The model under review builds one solid part; all positions refer to its coordinate system, in mm. A direction names the side the tool comes from. Round coordinates to 2 decimals unless told otherwise and drop trailing zeros. Write each loop counter-clockwise with the first axis right and the second up, starting at its lowest first coordinate (ties: lowest second). Pieces come first, ordered by that corner, then holes. Notation, with made-up numbers: (25.5, 3.25) - (48.5, 3.25) arc R9 ccw to (48.5, 16.25) - close; hole circle Ø9 at (50, 45). An arc over 180 degrees is marked (long way). Use one line per item in the form item = value.
from build123d import *

# Parameters (mm, degrees)
SKETCH1_W           = 7
SKETCH1_H           = 7
BOSS_EXTRUDE1_DEPTH = 3
CUT_EXTRUDE1_DEPTH  = 7
CUT_EXTRUDE2_DEPTH  = 11
SKETCH4_R           = 1.8
CUT_EXTRUDE3_DEPTH  = 0.8
CUT_EXTRUDE4_DEPTH  = 0.4


with BuildPart() as part:
    # Sketch1 → Boss-Extrude1 (new body)
    with BuildSketch(Plane(origin=(0, 0, 0), x_dir=(1, 0, 0), z_dir=(0, 1, 0))):
        with Locations((3.5, 3.5)):
            Rectangle(SKETCH1_W, SKETCH1_H)
    extrude(amount=BOSS_EXTRUDE1_DEPTH)

    # Sketch2 → Cut-Extrude1 (cut)
    with BuildSketch(Plane.XY):
        Polygon((0, 0), (0.7, 3), (0, 3), align=None)
        Polygon((7, 0), (6.3, 3), (7, 3), align=None)
    extrude(amount=-CUT_EXTRUDE1_DEPTH, mode=Mode.SUBTRACT)

    # Sketch3 → Cut-Extrude2 (cut)
    with BuildSketch(Plane(origin=(0, 0, 0), x_dir=(0, 0, -1), z_dir=(1, 0, 0))):
        Polygon((0, 0), (0.7, 3), (0, 3), align=None)
        Polygon((7, 3), (6.3, 3), (7, 0), align=None)
    extrude(amount=CUT_EXTRUDE2_DEPTH, mode=Mode.SUBTRACT)

    # Sketch4 → Cut-Extrude3 (cut)
    with BuildSketch(Plane.XZ):
        with Locations(Location((3.5, -3.5, 0), (0, 0, 270))):
            Circle(SKETCH4_R)
    extrude(amount=-CUT_EXTRUDE3_DEPTH, mode=Mode.SUBTRACT)

    # Sketch5 → Cut-Extrude4 (cut)
    with BuildSketch(Plane(origin=(0, 3, 0), x_dir=(1, 0, 0), z_dir=(0, 1, 0))):
        with BuildLine():
            Line((2.273436966, 1.766029319), (2.273436966, 5.266029319))
            Line((2.273436966, 5.266029319), (3.393128472, 5.266029319))
            add(Edge.make_bspline(
                [(3.393128472, 5.266029319), (3.443844607, 5.265973935), (3.540845243, 5.265868005), (3.679210782, 5.262924846), (3.803788221, 5.25875848), (3.914392667, 5.253569447), (4.011413307, 5.245826414), (4.094414918, 5.236860098), (4.163920155, 5.227214721), (4.20484973, 5.217233046), (4.223256678, 5.212744063)],
                knots=[0, 0, 0, 0, 1.460485487, 2.793352117, 3.985295279, 5.050041172, 5.981765236, 6.787433016, 7.454681457, 8, 8, 8, 8], degree=3))
            add(Edge.make_bspline(
                [(4.223256678, 5.212744063), (4.247733441, 5.205764794), (4.296314082, 5.191912581), (4.365914991, 5.162381864), (4.432999247, 5.128157338), (4.496724006, 5.087367889), (4.55730589, 5.040737674), (4.614924976, 4.988646969), (4.669888538, 4.930860625), (4.721436225, 4.867492795), (4.768647843, 4.798863014), (4.809450543, 4.724869813), (4.843634674, 4.645834805), (4.872758986, 4.562351928), (4.894247042, 4.473526111), (4.909284774, 4.379974525), (4.919752913, 4.281656252), (4.920494089, 4.214375246), (4.920872863, 4.179991659)],
                knots=[0, 0, 0, 0, 0.907145743, 1.80047177, 2.69161667, 3.591261238, 4.495029544, 5.415863088, 6.359363025, 7.337192411, 8.326890979, 9.326929023, 10.346104993, 11.395420813, 12.477187422, 13.601053412, 14.774031606, 16, 16, 16, 16], degree=3))
            add(Edge.make_bspline(
                [(4.920872863, 4.179991659), (4.919792601, 4.127776273), (4.917713038, 4.027258789), (4.894446409, 3.883154793), (4.858959078, 3.751525082), (4.807091778, 3.633637523), (4.743854765, 3.529029507), (4.674197894, 3.434725874), (4.594659983, 3.353569033), (4.508726287, 3.284249259), (4.417910076, 3.227520832), (4.326929468, 3.179160654), (4.234556815, 3.141979803), (4.171577346, 3.125779808), (4.140524306, 3.11779214)],
                knots=[0, 0, 0, 0, 1.312386234, 2.526415563, 3.661883817, 4.733421185, 5.753802465, 6.732107337, 7.675884281, 8.604170108, 9.50284679, 10.365392406, 11.194030444, 12, 12, 12, 12], degree=3))
            add(Edge.make_bspline(
                [(4.140524306, 3.11779214), (4.118360169, 3.113576), (4.071640813, 3.10468888), (3.997546708, 3.09583004), (3.916557837, 3.086024269), (3.828341085, 3.079628394), (3.733003173, 3.073638926), (3.63058112, 3.0708111), (3.521221299, 3.067404144), (3.44594969, 3.067342926), (3.407150908, 3.06731137)],
                knots=[0, 0, 0, 0, 0.735353946, 1.55003838, 2.431865514, 3.394945452, 4.432993119, 5.54609699, 6.735134699, 8, 8, 8, 8], degree=3))
            Line((3.407150908, 3.06731137), (2.946513889, 3.06731137))
            Line((2.946513889, 3.06731137), (2.946513889, 1.766029319))
            Line((2.946513889, 1.766029319), (2.273436966, 1.766029319))
        make_face()
        with BuildLine():
            Line((2.946513889, 4.682695986), (2.946513889, 3.650644704))
            Line((2.946513889, 3.650644704), (3.350360043, 3.650644704))
            add(Edge.make_bspline(
                [(3.350360043, 3.650644704), (3.385185484, 3.6506898), (3.451810934, 3.650776074), (3.547403676, 3.653872817), (3.633934317, 3.657652965), (3.711583659, 3.663909885), (3.779882991, 3.672156355), (3.839289696, 3.682020172), (3.889873011, 3.692605078), (3.94457198, 3.710145964), (4.003056114, 3.738525517), (4.065510296, 3.779314064), (4.120376221, 3.828081582), (4.166031944, 3.885357343), (4.202500757, 3.948994033), (4.228612454, 4.01833948), (4.245472753, 4.092244389), (4.247012787, 4.143440235), (4.24779594, 4.169474832)],
                knots=[0, 0, 0, 0, 1.411705958, 2.700771114, 3.876961699, 4.922619712, 5.858038221, 6.66485904, 7.363650596, 7.950905807, 8.989198271, 9.987739806, 10.967313358, 11.951275539, 12.944273208, 13.927870418, 14.946261014, 16, 16, 16, 16], degree=3))
            add(Edge.make_bspline(
                [(4.24779594, 4.169474832), (4.246693738, 4.201184565), (4.244556714, 4.262665556), (4.220991303, 4.350224748), (4.184632567, 4.429685776), (4.132649896, 4.498576249), (4.069856053, 4.556507472), (3.999278394, 4.604708309), (3.919409702, 4.638439621), (3.862884076, 4.65150926), (3.834134081, 4.658156723)],
                knots=[0, 0, 0, 0, 1.085904563, 2.105425768, 3.088705091, 4.068969419, 5.045188284, 6.010769642, 6.988240112, 8, 8, 8, 8], degree=3))
            add(Edge.make_bspline(
                [(3.834134081, 4.658156723), (3.821762302, 4.660135488), (3.794300788, 4.664527734), (3.748654162, 4.669111588), (3.694654197, 4.673280599), (3.6322358, 4.676703481), (3.561646383, 4.679379383), (3.482653109, 4.681724132), (3.395464024, 4.681912502), (3.334467378, 4.682427589), (3.302683761, 4.682695986)],
                knots=[0, 0, 0, 0, 0.564603001, 1.253243608, 2.066786758, 3.005752288, 4.070476343, 5.250658742, 6.567396469, 8, 8, 8, 8], degree=3))
            Line((3.302683761, 4.682695986), (2.946513889, 4.682695986))
        make_face(mode=Mode.SUBTRACT)
    extrude(amount=-CUT_EXTRUDE4_DEPTH, mode=Mode.SUBTRACT)


solid = part.part
(1) Add section B-B on z = -2.75. Write out the cut boundary in (x, y).
Geometry results:
outline = (0, 0) - (1.86, 0) - (1.86, 0.8) - (5.14, 0.8) - (5.14, 0) - (7, 0) - (6.3, 3) - (2.95, 3) - (2.95, 2.6) - (2.27, 2.6) - (2.27, 3) - (0.7, 3) - close
(2) To check wall thickness, follow L1, parallel to Z at x = 3.75, y = 0.55; L2, parallel to X at y = 0.65, z = -5; L3, parallel to X at y = 0.45, z = -3.5 (3 decimals). State the ranges of each line that lie inside material, in increasing order.
Geometry results:
L1 = -6.87 to -5.28, -1.72 to -0.13
L2 = 0.15 to 2.51, 4.49 to 6.85
L3 = 0.105 to 1.7, 5.3 to 6.895
(3) Add section A-A on y = 0.6. Write out the cut boundary in (x, z), then the cut area to 3 significant figures.
Geometry results:
outline = (0.14, -6.86) - (6.86, -6.86) - (6.86, -0.14) - (0.14, -0.14) - close; hole circle Ø3.6 at (3.5, -3.5)
area = 35.0 mm2
(4) Add section D-D on y = 1.35. Write out the cut boundary in (x, z) (3 decimals), then the cut area to 3 significant figures.
Geometry results:
outline = (0.315, -6.685) - (6.685, -6.685) - (6.685, -0.315) - (0.315, -0.315) - close
area = 40.6 mm2
(5) Insertion check: P1, Ø4, axis at x = 4, z = -3.5, coming from the +Y side; P2, Ø1.8, axis at x = 3.5, z = -3, coming from the -Y side. Each pin has a flat end and moves straight along its axis. Give the tip position at first contact, or say it passes through.
Geometry results:
P1 = 3
P2 = 0.8
(6) Add section C-C on x = 1. Write out the cut boundary in (y, z).
Geometry results:
outline = (0, -7) - (3, -6.3) - (3, -0.7) - (0, 0) - close
(7) Machinability: for faces 4 (the cylindrical face through (4.041, 0.394, -5.217)), 5 (the flat face through (3.5, 3, -2.9)), which of the approach directions +Z, -Z, +X, -X, +Y, -Y give a long, thin tool a straight path to every point of the face, cutting with its end or side? Answer none if there is none.
Geometry results:
face_4 = -Y
face_5 = +Z, -Z, +X, -X, +Y
(8) The part is to be moulded in two halves that separate along X. For faces 1 (the flat face through (0.345, 1.479, -3.451)), 2 (the flat face through (3.3, 2.6, -3.5)), 3 (the flat face through (4, 3, -4)), say which applies: +X half, -X half, draft (parallel to the pull), parting line (faces both ways), or undercut.
Geometry results:
face_1 = -X half
face_2 = undercut
face_3 = draft
